```python
from build123d import *

# Parameters (mm, degrees)
SKETCH2_R           = 2.05
SKETCH2_R_2         = 6.35
BOSS_EXTRUDE1_DEPTH = 6.35


with BuildPart() as part:
    # Sketch2 → Boss-Extrude1 (new body)
    with BuildSketch(Plane(origin=(0, 0, 0), x_dir=(1, 0, 0), z_dir=(0, 1, 0))):
        with BuildLine():
            ThreePointArc((-25.4, 22.86), (-24.656051224, 24.656051224), (-22.86, 25.4))
            Line((-22.86, 25.4), (22.86, 25.4))
            ThreePointArc((22.86, 25.4), (24.656051224, 24.656051224), (25.4, 22.86))
            Line((25.4, 22.86), (25.4, -22.86))
            ThreePointArc((25.4, -22.86), (24.656051224, -24.656051224), (22.86, -25.4))
            Line((22.86, -25.4), (-22.86, -25.4))
            ThreePointArc((-22.86, -25.4), (-24.656051224, -24.656051224), (-25.4, -22.86))
            Line((-25.4, -22.86), (-25.4, 22.86))
        make_face()
        with Locations(Location((-19.05, -19.05, 0), (0, 0, 270))):
            Circle(SKETCH2_R, mode=Mode.SUBTRACT)
        with Locations(Location((19.05, -19.05, 0), (0, 0, 270))):
            Circle(SKETCH2_R, mode=Mode.SUBTRACT)
        with Locations(Location((19.05, 19.05, 0), (0, 0, 270))):
            Circle(SKETCH2_R, mode=Mode.SUBTRACT)
        with Locations(Location((0, 0, 0), (0, 0, 270))):
            Circle(SKETCH2_R_2, mode=Mode.SUBTRACT)
        with Locations(Location((-19.05, 19.05, 0), (0, 0, 270))):
            Circle(SKETCH2_R, mode=Mode.SUBTRACT)
    extrude(amount=BOSS_EXTRUDE1_DEPTH)


solid = part.part
```
CAD build for the part. Positions are in the model's coordinates, mm. Round coordinates to 2 decimals unless told otherwise and drop trailing zeros. Order: outer loops, then holes, each group sorted by start corner. A loop starts at its lowest first (then second) coordinate and runs counter-clockwise, first axis right, second up. Notation, with made-up numbers: (40.5, -15) - (81.5, -15) arc R11 cw to (81.5, 2) - close; hole circle Ø11 at (34, -15). An arc over 180 degrees is marked (long way). Answer as CSV lines item,"result". Start each with the question number.
1. Pull direction Z, two halves, no side cores. Call faces 1 (the face through (-5, 0, -6)), 2 (the face through (19, 3, 17)), 3 (the face through (24.676, 3.131, 24.636)): +Z half, -Z half, draft (parallel to the pull), parting line (faces both ways), or undercut.
2. Saw through at B-B, the plane z = -19.05. Write the cut outline in (x, y), and give its area (3 significant figures).
3. Pin check, flat tip, straight feed: pin 1 (5.5 mm diameter, centred on x = 19.05, z = 19.05, fed in from +Y). Stop position of the tip, or through.
4. Saw through at C-C, the plane y = 1.25. Write the cut outline in (x, z).
5. Saw through at D-D, the plane x = 0. Write the cut outline in (y, z).
6. Drill centre lines: L1, parallel to X at y = 1.75, z = 19.05; L2, parallel to Z at x = 4.5, y = 1; L3, parallel to Z at x = 18, y = 6. Where is each one in solid material? Low to high. Write a range as [from, to].
7. Saw through at A-A, the plane x = -19.05. Write the cut outline in (y, z), and give its area (3 significant figures).
Model answer:
1,face 1,"draft"
1,face 2,"undercut"
1,face 3,"+Z half"
2,outline,"(-25.4, 0) - (-21.1, 0) - (-21.1, 6.35) - (-25.4, 6.35) - close; (-17, 0) - (17, 0) - (17, 6.35) - (-17, 6.35) - close; (21.1, 0) - (25.4, 0) - (25.4, 6.35) - (21.1, 6.35) - close"
2,area,"271 mm²"
3,pin 1,"stops at y = 6.35"
4,outline,"(-25.4, -22.86) arc R2.54 ccw to (-22.86, -25.4) - (22.86, -25.4) arc R2.54 ccw to (25.4, -22.86) - (25.4, 22.86) arc R2.54 ccw to (22.86, 25.4) - (-22.86, 25.4) arc R2.54 ccw to (-25.4, 22.86) - close; hole circle Ø4.1 at (-19.05, -19.05); hole circle Ø4.1 at (-19.05, 19.05); hole circle Ø12.7 at (0, 0); hole circle Ø4.1 at (19.05, -19.05); hole circle Ø4.1 at (19.05, 19.05)"
5,outline,"(0, -25.4) - (6.35, -25.4) - (6.35, -6.35) - (0, -6.35) - close; (0, 6.35) - (6.35, 6.35) - (6.35, 25.4) - (0, 25.4) - close"
6,L1,"x = [-25.4, -21.1], [-17, 17], [21.1, 25.4]"
6,L2,"z = [-25.4, -4.48], [4.48, 25.4]"
6,L3,"z = [-25.4, -20.81], [-17.29, 17.29], [20.81, 25.4]"
7,outline,"(0, -25.4) - (6.35, -25.4) - (6.35, -21.1) - (0, -21.1) - close; (0, -17) - (6.35, -17) - (6.35, 17) - (0, 17) - close; (0, 21.1) - (6.35, 21.1) - (6.35, 25.4) - (0, 25.4) - close"
7,area,"271 mm²"
